Read the model definition and answer for the solid it produces. Units are mm, in the model's axes. A direction names the side the tool comes from. Give positions to 0.01 mm unless a question says otherwise; leave off trailing zeros. Order: outer loops, then holes, each group sorted by start corner. A loop starts at its lowest first (then second) coordinate and runs counter-clockwise, first axis right, second up. Notation, with made-up numbers: M 85,51.5 L 134,51.5 A25 cw 134,84.5 Z; hole C 73,5.5 d8. An arc over 180 degrees is marked long. One line per item, written item: value. Start each with the question number.
Autodesk Inventor part; units mm, degrees
ref_plane "YZ Plane" through (0, 0, 0) normal (1, 0, 0) x (0, 1, 0)
ref_plane "XZ Plane" through (0, 0, 0) normal (0, 1, 0) x (-1, 0, 0)
ref_plane "XY Plane" through (0, 0, 0) normal (0, 0, 1) x (1, 0, 0)
sketch "Sketch1" plane through (0, 0, 0) normal (0, 0, 1) x (1, 0, 0)
  line L0 (-28.575, -28.575) -> (28.575, -28.575)
  line L1 (28.575, -28.575) -> (28.575, 28.575)
  line L2 (28.575, 28.575) -> (-28.575, 28.575)
  line L3 (-28.575, 28.575) -> (-28.575, -28.575)
  line L4 (-28.575, -28.575) -> (28.575, 28.575) construction
  line L5 (28.575, -28.575) -> (-28.575, 28.575) construction
  line L6 (-28.575, 0) -> (28.575, 0) construction
  line L7 (0, 28.575) -> (0, -28.575) construction
  circle A0 centre (-24.765, 24.765) radius 1.3
  circle A1 centre (24.765, 24.765) radius 1.3
  circle A2 centre (-24.765, -24.765) radius 1.3
  circle A3 centre (24.765, -24.765) radius 1.3
  circle A4 centre (0, -21) radius 1.3
  circle A5 centre (0, 21) radius 1.3
  line L8 (-12.5, 10) -> (12.5, 10)
  line L9 (12.5, 10) -> (12.5, -10)
  line L10 (12.5, -10) -> (-12.5, -10)
  line L11 (-12.5, -10) -> (-12.5, 10)
  line L12 (12.5, 10) -> (-12.5, -10) construction
  line L13 (12.5, -10) -> (-12.5, 10) construction
  point P0 (0, 0)
  point P1 (0, 0)
  dimension "d2" = 57.15
  dimension "d4" = 57.15
  dimension "d27" = 2.6
  dimension "d28" = 3.81
  dimension "d29" = 2.6
  dimension "d30" = 42
  dimension "d31" = 25
  dimension "d32" = 20
extrude "Extrusion1" add sketch "Sketch1" along normal blind 1.64
sketch "Sketch4" plane through (0, 0, 1.64) normal (0, 0, 1) x (1, 0, 0)
  line L0 (28.575, -28.575) -> (28.575, 28.575)
  line L1 (-28.575, 28.575) -> (-28.575, -28.575)
  line L2 (0, 0) -> (0, 45.0767)
  line L3 (21.035, 22.5) -> (26.035, 22.5)
  line L4 (26.035, 22.5) -> (26.035, -22.5)
  line L5 (26.035, -22.5) -> (21.035, -22.5)
  line L6 (21.035, -22.5) -> (21.035, 22.5)
  line L7 (-21.035, 22.5) -> (-26.035, 22.5)
  line L8 (-26.035, 22.5) -> (-26.035, -22.5)
  line L9 (-26.035, -22.5) -> (-21.035, -22.5)
  line L10 (-21.035, -22.5) -> (-21.035, 22.5)
  dimension "d21" = 2.54
  dimension "d22" = 45
  dimension "d23" = 5
  dimension "d24" = 22.5
extrude "Extrusion4" add sketch "Sketch4" along normal blind 5
properties part number "SFE-Host01" material "PCB(1)"
Q1. Each of these flat-tipped pins is pushed along its axis until it touches: pin 1 (2.5 mm diameter, centred on y = 4, z = 4, fed in from +X) (3 decimals); pin 2 (2 mm diameter, centred on x = 5, y = -10.5, fed in from +Z); pin 3 (2.5 mm diameter, centred on x = -23, z = 3.5, fed in from +Y). Where does it stop, or does it pass through?
Q2. Find section D-D, the plane y = 13. Give the vertices of the cut face in (x, z) (3 decimals).
Q3. Find section B-B, the plane y = 21. Give the vertices of the cut face in (x, z) (3 decimals).
Q4. Find section C-C, the plane z = 2.5. Give the vertices of the cut face in (x, y) (3 decimals).
Q5. Consider probe 1 along Y at (x, z) = (0, 0.3) (3 decimals); probe 2 along X at (y, z) = (-7, 3.25) (3 decimals); probe 3 along Z at (x, y) = (0.5, 25). Determine where each line is inside the solid, lowest interval first.
Q6. Determine the mould class of faces 5 (the cylindrical face through (-0.28, 22.27, 0.81)), 6 (the flat face through (-24, 0, 6.64)), 7 (the flat face through (0, -28.575, 1)) for opening direction Y: released by +Y, released by -Y, zero draft, split by the parting line, or undercut.
Q7. Find section A-A, the plane x = 0. Give the vertices of the cut face in (y, z) (3 decimals).
Q8. A tool of negligible diameter and unlimited length cuts with its end or side. For faces 1 (the flat face through (12.5, 0, 1)), 2 (the flat face through (-24, 22.5, 4)), 3 (the flat face through (24, -22.5, 4)), 4 (the flat face through (-26.035, 0, 4)), from which of +Z, -Z, +X, -X, +Y, -Y can it reach the whole face along a straight path? Write none if from no direction.
Evaluation:
1. pin 1: x = 26.035
1. pin 2: z = 1.64
1. pin 3: y = 22.5
2. outline: M -28.575,0 L 28.575,0 L 28.575,1.64 L 26.035,1.64 L 26.035,6.64 L 21.035,6.64 L 21.035,1.64 L -21.035,1.64 L -21.035,6.64 L -26.035,6.64 L -26.035,1.64 L -28.575,1.64 Z
3. outline: M -28.575,0 L -1.3,0 L -1.3,1.64 L -21.035,1.64 L -21.035,6.64 L -26.035,6.64 L -26.035,1.64 L -28.575,1.64 Z; M 1.3,0 L 28.575,0 L 28.575,1.64 L 26.035,1.64 L 26.035,6.64 L 21.035,6.64 L 21.035,1.64 L 1.3,1.64 Z
4. outline: M -26.035,-22.5 L -21.035,-22.5 L -21.035,22.5 L -26.035,22.5 Z; M 21.035,-22.5 L 26.035,-22.5 L 26.035,22.5 L 21.035,22.5 Z
5. probe 1: -28.575 to -22.3, -19.7 to -10, 10 to 19.7, 22.3 to 28.575
5. probe 2: -26.035 to -21.035, 21.035 to 26.035
5. probe 3: 0 to 1.64
6. face 5: undercut
6. face 6: zero draft
6. face 7: released by -Y
7. outline: M -28.575,0 L -22.3,0 L -22.3,1.64 L -28.575,1.64 Z; M -19.7,0 L -10,0 L -10,1.64 L -19.7,1.64 Z; M 10,0 L 19.7,0 L 19.7,1.64 L 10,1.64 Z; M 22.3,0 L 28.575,0 L 28.575,1.64 L 22.3,1.64 Z
8. face 1: +Z, -Z
8. face 2: +Z, +X, -X, +Y
8. face 3: +Z, +X, -X, -Y
8. face 4: +Z, -X, +Y, -Y
